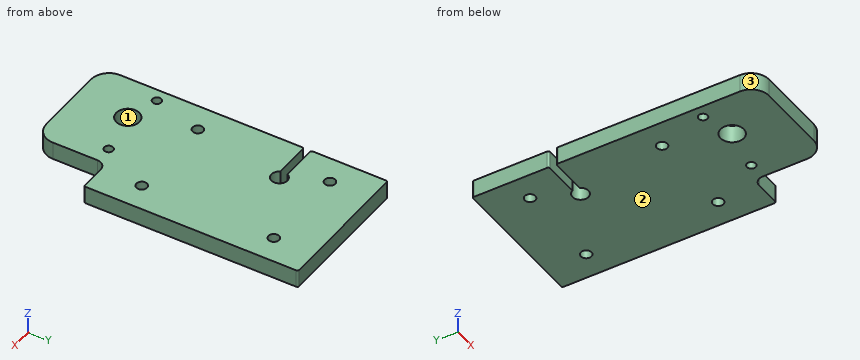
from build123d import *

# Parameters (mm, degrees)
SKETCH_R    = 3
SKETCH_R_2  = 2.5
SKETCH_R_3  = 6.5
PAD_DEPTH   = 10
FILLET_R    = 5
FILLET001_R = 1
FILLET002_R = 10


with BuildPart() as part:
    # Sketch → Pad (new body)
    with BuildSketch(Plane.XY):
        with BuildLine():
            ThreePointArc((-4.031129, -2), (4.5, 0), (-4.031129, 2))
            Line((-4.031129, 2), (-25, 2))
            Line((-25, 45), (-25, 2))
            Line((-25, 45), (55, 45))
            Line((55, 45), (55, -75))
            Line((35, -75), (55, -75))
            Line((35, -115), (35, -75))
            Line((-25, -115), (35, -115))
            Line((-25, -2), (-25, -115))
            Line((-4.031129, -2), (-25, -2))
        make_face()
        with Locations((-10, -52)):
            Circle(SKETCH_R, mode=Mode.SUBTRACT)
        with Locations((40, -52)):
            Circle(SKETCH_R, mode=Mode.SUBTRACT)
        with Locations((40, 22)):
            Circle(SKETCH_R, mode=Mode.SUBTRACT)
        with Locations((-10, 22)):
            Circle(SKETCH_R, mode=Mode.SUBTRACT)
        with Locations((25, -80)):
            Circle(SKETCH_R_2, mode=Mode.SUBTRACT)
        with Locations((-18, -80)):
            Circle(SKETCH_R_2, mode=Mode.SUBTRACT)
        with Locations((0, -85)):
            Circle(SKETCH_R_3, mode=Mode.SUBTRACT)
    extrude(amount=PAD_DEPTH)

    # Fillet
    fillet_edges = [part.edges().sort_by_distance(p)[0] for p in [
        (35, -75, 5),
    ]]
    fillet(fillet_edges, radius=FILLET_R)

    # Fillet001
    fillet001_edges = [part.edges().sort_by_distance(p)[0] for p in [
        (55, -75, 5),
        (55, 45, 5),
        (-25, 2, 5),
        (-25, -2, 5),
        (-25, 45, 5),
    ]]
    fillet(fillet001_edges, radius=FILLET001_R)

    # Fillet002
    fillet002_edges = [part.edges().sort_by_distance(p)[0] for p in [
        (-25, -115, 5),
        (35, -115, 5),
    ]]
    fillet(fillet002_edges, radius=FILLET002_R)


solid = part.part
The listing builds one solid part. Answer for the finished solid, in the listing's coordinates (mm). Face numbers are marked on the shaded views. Give positions to 0.01 mm unless a question says otherwise; leave off trailing zeros. Loops run counter-clockwise (first coordinate to the right, second up) from the corner with the lowest first, then second, coordinate; pieces in that order, holes last.
Item 1: Each of these flat-tipped pins is pushed along its axis until it touches: pin 1 Ø3 at (x, z) = (46.5, 3) entering from -Y; pin 2 Ø2 at (y, z) = (-79, 2) entering from +X; pin 3 Ø5 at (y, z) = (-92.5, 5.5) entering from +X; pin 4 Ø8 at (x, y) = (-10, -52) entering from -Z. Where does it stop, or does it pass through?
Derived:
pin 1: stops at y = -75
pin 2: stops at x = 35.42
pin 3: stops at x = 35
pin 4: stops at z = 0
Item 2: A cutting plane is placed at A-A (x = -10). Give the vertices of the cut face in (y, z).
Derived:
outline: (-115, 0) - (-55, 0) - (-55, 10) - (-115, 10) - close; (-49, 0) - (-2, 0) - (-2, 10) - (-49, 10) - close; (2, 0) - (19, 0) - (19, 10) - (2, 10) - close; (25, 0) - (45, 0) - (45, 10) - (25, 10) - close
Item 3: A cutting plane is placed at D-D (z = 4). Give the vertices of the cut face in (x, y).
Derived:
outline: (-25, -105) arc R10 ccw to (-15, -115) - (25, -115) arc R10 ccw to (35, -105) - (35, -80) arc R5 cw to (40, -75) - (54, -75) arc R1 ccw to (55, -74) - (55, 44) arc R1 ccw to (54, 45) - (-24, 45) arc R1 ccw to (-25, 44) - (-25, 3) arc R1 ccw to (-24, 2) - (-4.03, 2) arc R4.5 cw (long way) to (-4.03, -2) - (-24, -2) arc R1 ccw to (-25, -3) - close; hole circle Ø5 at (-18, -80); hole circle Ø6 at (-10, -52); hole circle Ø6 at (-10, 22); hole circle Ø13 at (0, -85); hole circle Ø5 at (25, -80); hole circle Ø6 at (40, -52); hole circle Ø6 at (40, 22)
Item 4: A cutting plane is placed at B-B (x = 0). Give the vertices of the cut face in (y, z).
Derived:
outline: (-115, 0) - (-91.5, 0) - (-91.5, 10) - (-115, 10) - close; (-78.5, 0) - (-4.5, 0) - (-4.5, 10) - (-78.5, 10) - close; (4.5, 0) - (45, 0) - (45, 10) - (4.5, 10) - close
Item 5: A cutting plane is placed at C-C (y = -52). Give the vertices of the cut face in (x, z), then the cut area to 3 significant figures.
Derived:
outline: (-25, 0) - (-13, 0) - (-13, 10) - (-25, 10) - close; (-7, 0) - (37, 0) - (37, 10) - (-7, 10) - close; (43, 0) - (55, 0) - (55, 10) - (43, 10) - close
area: 680 mm2
Item 6: Determine the mould class of the marked faces 1, 2 and 3 for opening direction Y: +Y half, -Y half, draft (parallel to the pull), parting line (faces both ways), or undercut.
Derived:
face 1: undercut
face 2: draft
face 3: -Y half
Item 7: Find the intervals of material crossed by line 1 along Y through (x, z) = (-10, 2.25); line 2 along Y through (x, z) = (0, 8); line 3 along Y through (x, z) = (42.5, 4.25), in increasing order.
Derived:
line 1: y = -115 to -55, -49 to -2, 2 to 19, 25 to 45
line 2: y = -115 to -91.5, -78.5 to -4.5, 4.5 to 45
line 3: y = -75 to -53.66, -50.34 to 20.34, 23.66 to 45
